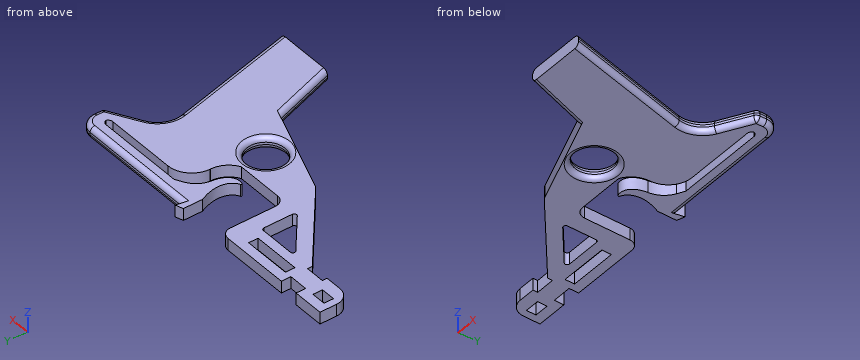
from build123d import *

# Parameters (mm, degrees)
F0_W     = 7.62
F0_H     = 5.08
F0_W_2   = 25.4
F0_R     = 10.16
F1_DEPTH = 6.35
F2_R     = 2.54


with BuildPart() as f1:
    # F0 (on Top) → F1 (new body)
    with BuildSketch(Plane.XY):
        with BuildLine():
            Line((-31.6706262529, -6.5881243579), (15.2908454792, -6.5881243579))
            ThreePointArc((15.2908454792, -6.5881243579), (16.7968803502, -7.0827737847), (17.7163331065, -8.374062179))
            ThreePointArc((17.7163331065, -8.374062179), (16.7968803502, -9.6653505732), (15.2908454792, -10.16))
            Line((15.2908454792, -10.16), (-22.8091545208, -10.16))
            ThreePointArc((-22.8091545208, -10.16), (-31.7894106419, -13.8797438789), (-35.5091545208, -22.86))
            Line((-35.5091545208, -22.86), (-35.5091545208, -23.067451765))
            ThreePointArc((-35.5091545208, -23.067451765), (-37.3281393906, -29.6167654494), (-42.2640379439, -34.29))
            Line((-42.2640379439, -34.29), (-67.31, -34.29))
            ThreePointArc((-67.31, -34.29), (-70.9021024484, -32.8021024484), (-72.39, -29.21))
            Line((-72.39, -29.21), (-72.39, -5.08))
            ThreePointArc((-72.39, -5.08), (-73.8778975516, -1.4878975516), (-77.47, 0))
            Line((-77.47, 0), (-114.3, 0))
            Line((-114.3, 0), (-114.3, -5.08))
            Line((-114.3, -5.08), (-124.46, -5.08))
            Line((-124.46, -5.08), (-124.46, 0))
            Line((-124.46, 0), (-140.97, 0))
            Line((-140.97, 0), (-140.97, -8.89))
            ThreePointArc((-140.97, -8.89), (-138.7381536726, -14.2781536726), (-133.35, -16.51))
            Line((-133.35, -16.51), (-124.46, -16.51))
            Line((-124.46, -16.51), (-124.46, -13.97))
            Line((-124.46, -13.97), (-114.3, -13.97))
            Line((-114.3, -13.97), (-114.3, -16.51))
            Line((-114.3, -16.51), (-73.1955929906, -50.0475420508))
            ThreePointArc((-73.1955929906, -50.0475420508), (-72.1633213981, -50.756926583), (-71.0287858488, -51.2876243715))
            Line((-71.0287858488, -51.2876243715), (-24.3288669735, -68.6128414369))
            Line((-24.3288669735, -68.6128414369), (-12.7, -103.0557602644))
            Line((-12.7, -103.0557602644), (19.05, -103.0557602644))
            Line((19.05, -103.0557602644), (2.3547967276, -36.4372610145))
            ThreePointArc((2.3547967276, -36.4372610145), (3.0065319132, -28.3336286948), (8.4393105622, -22.2856098724))
            Line((8.4393105622, -22.2856098724), (24.1577511408, -13.4286290107))
            ThreePointArc((24.1577511408, -13.4286290107), (25.1038731102, -12.4972467832), (25.4508454792, -11.2157516369))
            Line((25.4508454792, -11.2157516369), (25.4508454792, -7.62))
            ThreePointArc((25.4508454792, -7.62), (23.2189991518, -2.2318463274), (17.8308454792, 0))
            Line((17.8308454792, 0), (12.0385419577, 0))
            Line((12.0385419577, 0), (-46.4872904122, 0))
            Line((-46.4872904122, 0), (-45.8256908553, 3.752117539))
            Line((-45.8256908553, 3.752117539), (-49.8210415244, 2.54))
            Line((-49.8210415244, 2.54), (-49.8210415244, 0))
            Line((-49.8210415244, 0), (-49.8210415244, -7.5935418718))
            add(Edge.make_bspline(
                [(-49.8210415244, -7.5935418718), (-44.485431179, -18.5982405148), (-47.5559489311, -24.9495477887), (-51.5999285014, -26.6474626741)],
                knots=[0, 0, 0, 0, 17.7354547772, 17.7354547772, 17.7354547772, 17.7354547772], degree=3))
            ThreePointArc((-51.5999285014, -26.6474626741), (-51.8920952454, -27.1191706564), (-51.5419420272, -27.5495920205))
            add(Edge.make_bspline(
                [(-42.1931219537, -18.7228273079), (-42.6397200116, -23.7693324215), (-45.6204470158, -29.1828876463), (-51.5419420272, -27.5495920205)],
                knots=[5.2109253832, 5.2109253832, 5.2109253832, 5.2109253832, 16.5043202027, 16.5043202027, 16.5043202027, 16.5043202027], degree=3))
            ThreePointArc((-42.1931219537, -18.7228273079), (-40.130905812, -12.8297269732), (-35.5096463796, -8.6314739761))
            Line((-35.5096463796, -8.6314739761), (-31.6706262529, -6.5881243579))
        make_face()
        with BuildLine():
            Line((-83.0959535938, -32.5987200656), (-101.7744590691, -17.3587200656))
            ThreePointArc((-101.7744590691, -17.3587200656), (-102.1679568897, -15.9485577312), (-100.9715862663, -15.1047001153))
            Line((-100.9715862663, -15.1047001153), (-82.2930807911, -15.1047001153))
            ThreePointArc((-82.2930807911, -15.1047001153), (-81.3950551789, -15.4766745032), (-81.0230807911, -16.3747001153))
            Line((-81.0230807911, -16.3747001153), (-81.0230807911, -31.6147001153))
            ThreePointArc((-81.0230807911, -31.6147001153), (-81.74844718, -32.7619900655), (-83.0959535938, -32.5987200656))
        make_face(mode=Mode.SUBTRACT)
        with Locations((-133.35, -7.62)):
            Rectangle(F0_W, F0_H, mode=Mode.SUBTRACT)
        with Locations((-97.79, -7.62)):
            Rectangle(F0_W_2, F0_H, mode=Mode.SUBTRACT)
        with Locations((-40.8155657351, -48.4425649047)):
            Circle(F0_R, mode=Mode.SUBTRACT)
        with BuildLine():
            ThreePointArc((17.8308454792, -9.1281243579), (17.8020542094, -8.7467705677), (17.7163331065, -8.374062179))
            ThreePointArc((17.7163331065, -8.374062179), (17.8020542094, -8.0013537902), (17.8308454792, -7.62))
            Line((17.8308454792, -7.62), (17.8308454792, -9.1281243579))
        make_face(mode=Mode.SUBTRACT)
        with BuildLine():
            ThreePointArc((17.8308454792, -7.62), (17.8020542094, -8.0013537902), (17.7163331065, -8.374062179))
            ThreePointArc((17.7163331065, -8.374062179), (17.8020542094, -8.7467705677), (17.8308454792, -9.1281243579))
            Line((17.8308454792, -9.1281243579), (17.8308454792, -7.62))
        make_face()
    extrude(amount=F1_DEPTH)

    # F2
    f2_edges = [f1.edges().sort_by_distance(p)[0] for p in [
        (-18.514433, -85.834301, 6.35),
        (-18.514433, -85.834301, 0),
        (-50.975566, -48.442565, 6.35),
        (-50.975566, -48.442565, 0),
        (10.702398, -69.746511, 6.35),
        (10.702398, -69.746511, 0),
        (3.006532, -28.333629, 0),
        (3.006532, -28.333629, 6.35),
        (16.298531, -17.857119, 0),
        (16.298531, -17.857119, 6.35),
        (25.103873, -12.497247, 0),
        (25.103873, -12.497247, 6.35),
        (25.450845, -9.417876, 0),
        (25.450845, -9.417876, 6.35),
        (23.218999, -2.231846, 0),
        (23.218999, -2.231846, 6.35),
        (-14.328222, 0, 0),
        (-14.328222, 0, 6.35),
    ]]
    fillet(f2_edges, radius=F2_R)


solid = f1.part
Model file for the job. Use its own axes, mm. Give positions to 0.01 mm unless a question says otherwise; leave off trailing zeros. Order: outer loops, then holes, each group sorted by start corner. A loop starts at its lowest first (then second) coordinate and runs counter-clockwise, first axis right, second up. Notation, with made-up numbers: (-33, 55.5) - (6, 55.5) arc R23 ccw to (6, 74.5) - close; hole circle Ø5 at (16, -3.5). An arc over 180 degrees is marked (long way). One line per item, written item: value.
Item 1: Slice it at A-A (x = -98.5). List the corners of the cut face in (y, z), then the cut area to 3 significant figures.
Response values:
outline: (-29.4, 0) - (-20.03, 0) - (-20.03, 6.35) - (-29.4, 6.35) - close; (-15.1, 0) - (-10.16, 0) - (-10.16, 6.35) - (-15.1, 6.35) - close; (-5.08, 0) - (0, 0) - (0, 6.35) - (-5.08, 6.35) - close
area: 123 mm2
Item 2: Slice it at B-B (z = 1.25). Give the number of separate pieces and of enclosed holes in the cut face, then the cut area to 3 significant figures.
Response values:
separate pieces: 1
enclosed holes: 4
area: 6,150 mm2
Item 3: Slice it at C-C (x = -55.5). List the corners of the cut face in (y, z), then the cut area to 3 significant figures.
Response values:
outline: (-57.05, 0) - (-34.29, 0) - (-34.29, 6.35) - (-57.05, 6.35) - close
area: 145 mm2
Item 4: Pin check, flat tips, straight feed: pin 1 Ø18.5 at (x, y) = (-40.82, -48.44) entering from -Z; pin 2 Ø3 at (x, z) = (-135, 3.5) entering from +Y; pin 3 Ø3 at (y, z) = (-19.5, 3) entering from +X; pin 4 Ø1 at (x, z) = (-46.5, 1) entering from -Y. Stop position of each tip, or through.
Response values:
pin 1: through
pin 2: y = 0
pin 3: x = 16.04
pin 4: y = -60.57
Item 5: Wall check: line 1 (X direction, y = -32, z = 6); line 2 (X direction, y = -22, z = 2.5); line 3 (Y direction, x = -5.5, z = 2.75). Give the ranges that are in metal, low to high.
Response values:
line 1: -95.32 to -83.83, -81.08 to -71.56, -39.18 to 0.79
line 2: -107.57 to -96.09, -81.02 to -72.39, -47.55 to -42.85, -35.48 to 8.95
line 3: -103.06 to -10.16, -6.59 to 0
